```python
from build123d import *

# Parameters (mm, degrees)
SKETCH2_W                = 120
SKETCH2_H                = 110
BOSS_EXTRUDE1_DEPTH      = 80
CUT_EXTRUDE1_DEPTH       = 161.930246459
SKETCH6_R                = 2
SKETCH6_W                = 10
SKETCH6_H                = 5
CUT_EXTRUDE4_DEPTH       = 14
CUT_EXTRUDE6_DEPTH       = 161.930246459
CUT_EXTRUDE8_DEPTH       = 120
BOSS_EXTRUDE11_DEPTH     = 55
BOSS_EXTRUDE12_DEPTH     = 55
SKETCH17_W               = 10
SKETCH17_H               = 5
BOSS_EXTRUDE13_DEPTH     = 7.333333
CUT_EXTRUDE9_DEPTH       = 161.930246459
BOSS_EXTRUDE14_DEPTH     = 20
SKETCH20_W               = 17.446322517
SKETCH20_H               = 1
BOSS_EXTRUDE15_DEPTH     = 5
BOSS_EXTRUDE16_DEPTH     = 1
CUT_EXTRUDE10_DEPTH      = 30
CUT_EXTRUDE12_DEPTH      = 30
FILLET1_R                = 5
FILLET2_R                = 5
FILLET3_R                = 5
CUT_EXTRUDE13_REACH      = 123.365
SKETCH25_R               = 5
CUT_EXTRUDE14_START      = -6.666667
SKETCH26_W               = 10
SKETCH26_H               = 6
CUT_EXTRUDE14_DEPTH      = 6.666667
SKETCH30_W               = 10
SKETCH30_H               = 14
CUT_EXTRUDE16_DEPTH      = 4
CUT_EXTRUDE18_DEPTH      = 2
CUT_EXTRUDE18_DEPTH_BACK = 1
SKETCH31_W               = 10
SKETCH31_H               = 14.8
SKETCH32_W               = 10
SKETCH32_H               = 7.905630189
BOSS_EXTRUDE18_DEPTH     = 5
CUT_EXTRUDE19_DEPTH      = 114.367474283
CUT_EXTRUDE19_DEPTH_BACK = 114.367474283


with BuildPart() as part:
    # Sketch2 → Boss-Extrude1 (new body)
    with BuildSketch(Plane(origin=(0, 0, 0), x_dir=(1, 0, 0), z_dir=(0, 1, 0))):
        with Locations((27.236913342, 16.404091096)):
            Rectangle(SKETCH2_W, SKETCH2_H)
    extrude(amount=BOSS_EXTRUDE1_DEPTH)

    # Sketch3 → Cut-Extrude1 (cut, through all)
    with BuildSketch(Plane(origin=(87.236913342, 0, 0), x_dir=(0, 0, -1), z_dir=(1, 0, 0))):
        Polygon((-38.595908904, 80), (41.404091096, 80), (-38.595908904, 20), align=None)
    extrude(amount=-CUT_EXTRUDE1_DEPTH, mode=Mode.SUBTRACT)

    # Sketch6 → Cut-Extrude4 (cut)
    with BuildSketch(Plane(origin=(0, 31.326036274, 23.494527206), x_dir=(1, 0, 0), z_dir=(0, 0.8, 0.6))):
        with Locations(Location((9.736913342, 66.123272877, 0), (0, 0, 270))):
            Circle(SKETCH6_R)
        with BuildLine():
            ThreePointArc((31.736913342, 74.123272877), (30.418893857, 77.305253392), (27.236913342, 78.623272877))
            Line((27.236913342, 78.623272877), (27.236913342, 69.623272877))
            ThreePointArc((27.236913342, 69.623272877), (30.418893857, 70.941292361), (31.736913342, 74.123272877))
        make_face()
        with BuildLine():
            Line((27.236913342, 69.623272877), (27.236913342, 78.623272877))
            ThreePointArc((27.236913342, 78.623272877), (22.736913342, 74.123272877), (27.236913342, 69.623272877))
        make_face()
        with Locations(Location((44.736913342, 66.123272877, 0), (0, 0, 270))):
            Circle(SKETCH6_R)
        with Locations((27.236913342, -5.376727123)):
            Rectangle(SKETCH6_W, SKETCH6_H)
    extrude(amount=-CUT_EXTRUDE4_DEPTH, mode=Mode.SUBTRACT)

    # Sketch8 → Cut-Extrude6 (cut, through all)
    with BuildSketch(Plane(origin=(87.236913342, 0, 0), x_dir=(0, 0, -1), z_dir=(1, 0, 0))):
        Polygon((41.904091096, 78.5), (12.704091096, 56.6), (51.404091096, 5), (66.404091096, 5), (66.404091096, 78.5), align=None)
    extrude(amount=-CUT_EXTRUDE6_DEPTH, mode=Mode.SUBTRACT)

    # Sketch12 → Cut-Extrude8 (cut)
    with BuildSketch(Plane(origin=(87.236913342, 0, 0), x_dir=(0, 0, -1), z_dir=(1, 0, 0))):
        Polygon((-25.795908904, 10), (-25.795908904, 27.725), (-38.595908904, 18.125), (-38.595908904, 2), align=None)
    extrude(amount=-CUT_EXTRUDE8_DEPTH, mode=Mode.SUBTRACT)

    # Sketch13 → Boss-Extrude11 (add)
    with BuildSketch(Plane(origin=(87.236913342, 0, 0), x_dir=(0, 0, -1), z_dir=(1, 0, 0))):
        Polygon((-38.595908904, 18.125), (-25.795908904, 27.725), (-25.795908904, 10), (-38.595908904, 2), align=None)
    extrude(amount=-BOSS_EXTRUDE11_DEPTH)

    # Sketch14 → Boss-Extrude12 (add)
    with BuildSketch(Plane.ZY.offset(32.763086658)):
        Polygon((38.595908904, 18.125), (25.795908904, 27.725), (25.795908904, 10), (38.595908904, 2), align=None)
    extrude(amount=-BOSS_EXTRUDE12_DEPTH)

    # Sketch17 → Boss-Extrude13 (add)
    with BuildSketch(Plane(origin=(0, 20.126036274, 15.094527206), x_dir=(1, 0, 0), z_dir=(0, 0.8000000000000005, 0.5999999999999995))):
        with Locations((27.236913342, -5.376727123)):
            Rectangle(SKETCH17_W, SKETCH17_H)
    extrude(amount=BOSS_EXTRUDE13_DEPTH)

    # Sketch18 → Cut-Extrude9 (cut, through all)
    with BuildSketch(Plane(origin=(87.236913342, 0, 0), x_dir=(0, 0, -1), z_dir=(1, 0, 0))):
        Polygon((51.404091096, 5), (14.804111641, 53.799972607), (-16.825372102, 29.858521527), (-16.825372102, 5), align=None)
    extrude(amount=-CUT_EXTRUDE9_DEPTH, mode=Mode.SUBTRACT)

    # Sketch19 → Boss-Extrude14 (add)
    with BuildSketch(Plane.XY.offset(38.595908904)):
        Polygon((17.236913342, 0), (37.236913342, 0), (37.236913342, 7), (35.9600746, 7), (35.9600746, 2), (18.513752083, 2), (18.513752083, 7), (17.236913342, 7), align=None)
    extrude(amount=BOSS_EXTRUDE14_DEPTH)

    # Sketch20 → Boss-Extrude15 (add)
    with BuildSketch(Plane(origin=(0, 2, 0), x_dir=(1, 0, 0), z_dir=(0, 1, 0))):
        with Locations((27.236913342, -58.095908904)):
            Rectangle(SKETCH20_W, SKETCH20_H)
    extrude(amount=BOSS_EXTRUDE15_DEPTH)

    # Sketch21 → Boss-Extrude16 (add)
    with BuildSketch(Plane(origin=(0, 31.326036274, 23.494527206), x_dir=(1, 0, 0), z_dir=(0, 0.8, 0.6))):
        with BuildLine():
            Line((20.612624354, 71.860797373), (21.371214726, 75.385643561))
            ThreePointArc((21.371214726, 75.385643561), (27.236913342, 80.123272877), (33.102611958, 75.385643561))
            Line((33.102611958, 75.385643561), (33.86120233, 71.860797373))
            ThreePointArc((33.86120233, 71.860797373), (34.142346815, 72.976543378), (34.236913342, 74.123272877))
            ThreePointArc((34.236913342, 74.123272877), (34.197727754, 74.862909761), (34.080609707, 75.594265758))
            ThreePointArc((34.080609707, 75.594265758), (27.236913342, 81.123272877), (20.393216976, 75.594265758))
            ThreePointArc((20.393216976, 75.594265758), (20.248969874, 73.71260746), (20.612624354, 71.860797373))
        make_face()
        with BuildLine():
            ThreePointArc((34.236913342, 74.123272877), (34.142346815, 72.976543378), (33.86120233, 71.860797373))
            Line((33.86120233, 71.860797373), (51.236913342, -8.876727123))
            Line((51.236913342, -8.876727123), (52.236913342, -8.876727123))
            Line((52.236913342, -8.876727123), (34.080609707, 75.594265758))
            ThreePointArc((34.080609707, 75.594265758), (34.197727754, 74.862909761), (34.236913342, 74.123272877))
        make_face()
        with BuildLine():
            Line((3.236913342, -8.876727123), (20.612624354, 71.860797373))
            ThreePointArc((20.612624354, 71.860797373), (20.248969874, 73.71260746), (20.393216976, 75.594265758))
            Line((20.393216976, 75.594265758), (2.236913342, -8.876727123))
            Line((2.236913342, -8.876727123), (3.236913342, -8.876727123))
        make_face()
    extrude(amount=BOSS_EXTRUDE16_DEPTH)

    # Sketch23 → Cut-Extrude10 (cut)
    with BuildSketch(Plane(origin=(87.236913342, 0, 0), x_dir=(0, 0, -1), z_dir=(1, 0, 0))):
        Polygon((-38.595908904, 0), (-38.595908904, 20), (41.404091096, 80), (71.404091096, 80), (71.404091096, 0), align=None)
    extrude(amount=-CUT_EXTRUDE10_DEPTH, mode=Mode.SUBTRACT)

    # Sketch24 → Cut-Extrude12 (cut)
    with BuildSketch(Plane.ZY.offset(32.763086658)):
        Polygon((-71.404091096, 80), (-41.404091096, 80), (38.595908904, 20), (38.595908904, 0), (-71.404091096, 0), align=None)
    extrude(amount=-CUT_EXTRUDE12_DEPTH, mode=Mode.SUBTRACT)

    # Fillet1
    fillet1_edges = [part.edges().sort_by_distance(p)[0] for p in [
        (27.236913342, 80, -71.404091096),
    ]]
    fillet(fillet1_edges, radius=FILLET1_R)

    # Fillet2
    fillet2_edges = [part.edges().sort_by_distance(p)[0] for p in [
        (57.236913342, 10, 38.595908904),
        (-2.763086658, 10, 38.595908904),
    ]]
    fillet(fillet2_edges, radius=FILLET2_R)

    # Fillet3
    fillet3_edges = [part.edges().sort_by_distance(p)[0] for p in [
        (57.236913342, 17.429260763, 16.825372102),
        (-2.763086658, 17.429260763, 16.825372102),
    ]]
    fillet(fillet3_edges, radius=FILLET3_R)

    # Sketch25 → Cut-Extrude13 (cut, up to next)
    with BuildSketch(Plane(origin=(0, 31.326036274, 23.494527206), x_dir=(1, 0, 0), z_dir=(0, 0.8, 0.6)), mode=Mode.PRIVATE) as cut_extrude13_sk1:
        with Locations(Location((27.236913342, 74.123272877, 0), (0, 0, 270))):
            Circle(SKETCH25_R)
    cut_extrude13_tool1 = extrude(cut_extrude13_sk1.sketch, amount=-CUT_EXTRUDE13_REACH, mode=Mode.PRIVATE) & part.part
    add(cut_extrude13_tool1.solids().sort_by_distance((27.236913, 75.8, -35.804091))[0], mode=Mode.SUBTRACT)

    # Sketch26 → Cut-Extrude14 (cut)
    with BuildSketch(Plane(origin=(0, 31.326036274, 23.494527206), x_dir=(1, 0, 0), z_dir=(0, 0.8, 0.6)).offset(CUT_EXTRUDE14_START)):
        with Locations((27.236913342, -4.876727123)):
            Rectangle(SKETCH26_W, SKETCH26_H)
    extrude(amount=CUT_EXTRUDE14_DEPTH, mode=Mode.SUBTRACT)

    # Sketch30 → Cut-Extrude16 (cut)
    with BuildSketch(Plane.XY.offset(25.795908904)):
        with Locations((27.236913342, 17)):
            Rectangle(SKETCH30_W, SKETCH30_H)
    extrude(amount=-CUT_EXTRUDE16_DEPTH, mode=Mode.SUBTRACT)

    # Sketch31 → Cut-Extrude18 (cut, two sides: drawn at the far end of the back side and taken through both)
    with BuildSketch(Plane.XY.offset(21.795908904).offset(-CUT_EXTRUDE18_DEPTH_BACK)):
        with Locations((27.236913342, 17.4)):
            Rectangle(SKETCH31_W, SKETCH31_H)
    extrude(amount=CUT_EXTRUDE18_DEPTH + CUT_EXTRUDE18_DEPTH_BACK, mode=Mode.SUBTRACT)

    # Sketch32 → Boss-Extrude18 (add)
    with BuildSketch(Plane(origin=(0, 18.784678159, 11.740423849), x_dir=(1, 0, 0), z_dir=(0, 0.8479983040050879, 0.5299989400031804))):
        with Locations((27.236913342, -12.622082506)):
            Rectangle(SKETCH32_W, SKETCH32_H)
    extrude(amount=-BOSS_EXTRUDE18_DEPTH)

    # Sketch36 → Cut-Extrude19 (cut, two sides: drawn at the far end of the back side and taken through both)
    with BuildSketch(Plane(origin=(32.236913342, 0, 0), x_dir=(0, 0, -1), z_dir=(1, 0, 0)).offset(-CUT_EXTRUDE19_DEPTH_BACK)):
        Polygon((-16.441953212, 9.9499841), (-16.825372102, 10.563454323), (-16.825372102, 9.710347294), align=None)
    extrude(amount=CUT_EXTRUDE19_DEPTH + CUT_EXTRUDE19_DEPTH_BACK, mode=Mode.SUBTRACT)


solid = part.part
```
Verification items for the finished model (mm, model axes). A direction names the side the tool comes from. Coordinates: 2 decimals unless noted, no trailing zeros. Write each loop counter-clockwise with the first axis right and the second up, starting at its lowest first coordinate (ties: lowest second). Pieces come first, ordered by that corner, then holes. Notation, with made-up numbers: (89, -31.75) - (103, -31.75) arc R17 cw to (103, -25.75) - close; hole circle Ø1 at (25.5, -2.75). An arc over 180 degrees is marked (long way). One line per question, with ' | ' between items. Start each with the question number.
1. Draft check along Z on faces 5 (the flat face through (27, 37, -71.404)), 6 (the flat face through (27.17, 7.64, 29.57)), 7 (the flat face through (27, 7, 58)). Enter one of: released by +Z, released by -Z, zero draft, split by the parting line, or undercut.
2. Section check A-A (z = -61). Enter the section's corners in (x, y).
3. Section check C-C (x = 15). Enter the section's corners in (y, z).
4. Section check B-B (y = 63.5). Enter the section's corners in (x, z).
5. Material ranges on line 1 along Z through (x, y) = (43, 7); line 2 along Y through (x, z) = (26.5, -50); line 3 along Y through (x, z) = (29, -16.5), recorded low to high.
6. Gauge pin test, flat ends, axial feed: P1, Ø3.5, axis at y = 2.5, z = 53, coming from the +X side; P2, Ø4, axis at x = 5, z = -6, coming from the +Y side; P3, Ø4, axis at x = 42, y = 66, coming from the +Z side. Record the tip position at first contact, or that the pin passes through.
7. Section check D-D (z = 41.5). Enter the section's corners in (x, y), plus the area to 3 significant figures.
8. Access from +Z, -Z, +X, -X, +Y, -Y to the whole of each face (thin tool, end or side, straight path). Record for faces 1 (the flat face through (28, 78.5, -54)), 2 (the cylindrical face through (-1.34, 17.6, 18.33)), 3 (the flat face through (22.237, 17, 29)), 4 (the cylindrical face through (27.4, 80.4, -41.1)).
Computed values:
1) face 5: released by -Z | face 6: undercut | face 7: zero draft
2) outline: (-2.76, 0) - (57.24, 0) - (57.24, 5) - (-2.76, 5) - close; (-2.76, 78.5) - (57.24, 78.5) - (57.24, 80) - (-2.76, 80) - close
3) outline: (0, -71.4) - (75, -71.4) arc R5 ccw to (80, -66.4) - (80, -41.4) - (61.63, -16.91) - (62.43, -16.31) - (59.59, -12.53) - (58.79, -13.13) - (20, 38.6) - (0, 38.6) - close; hole (5, -66.4) - (78.5, -66.4) - (78.5, -41.9) - (56.6, -12.7) - (53.8, -14.8) - (29.86, 16.83) - (5, 16.83) - close
4) outline: (-2.76, -71.4) - (57.24, -71.4) - (57.24, -66.4) - (-2.76, -66.4) - close; (-2.76, -21.9) - (57.24, -21.9) - (57.24, -19.4) - (38.8, -19.4) - (39.09, -17.74) - (38.07, -17.74) - (37.79, -19.4) - (16.69, -19.4) - (16.4, -17.74) - (15.38, -17.74) - (15.67, -19.4) - (-2.76, -19.4) - close
5) line 1: -71.4 to -66.4, 16.83 to 38.6 | line 2: 0 to 5, 78.5 to 80 | line 3: 0 to 5, 59.45 to 61.32
6) P1: x = 37.24 | P2: y = 54.95 | P3: z = -20.07
7) outline: (17.24, 0) - (37.24, 0) - (37.24, 7) - (35.96, 7) - (35.96, 2) - (18.51, 2) - (18.51, 7) - (17.24, 7) - close | area: 52.8 mm²
8) face 1: +X, -X | face 2: -X | face 3: none | face 4: +Y
